Part model, mm, in its own coordinate system. Face numbers are marked on the shaded views. Round coordinates to 2 decimals unless told otherwise and drop trailing zeros. Write each loop counter-clockwise with the first axis right and the second up, starting at its lowest first coordinate (ties: lowest second). Pieces come first, ordered by that corner, then holes. Notation, with made-up numbers: M 67.5,-17 L 112.5,-17 A18 cw 112.5,-12 Z; hole C 25,2.5 d11. An arc over 180 degrees is marked long. Use a Markdown table: item, result. Add a question column.
1) Wall check: probe 1 along X at (y, z) = (0, 1.35); probe 2 along X at (y, z) = (-5.25, 0.75). Give the ranges that are in metal, low to high.
2) Two-plate mould, pull along Y, no slides. Class the marked faces 1, 2 and 3: released by +Y, released by -Y, zero draft, split by the parting line, or undercut.
3) Slice it at C-C on z = -1.05. Write the cut outline in (x, y), plus the area to 3 significant figures.
4) Drop flat-ended pins along their axis: P1, Ø7, axis at x = 0, y = 0, coming from the +Z side; P2, Ø2, axis at y = 4.5, z = 0, coming from the +X side; P3, Ø3, axis at x = -6, z = -2, coming from the -Y side. Give the stop position or say it passes through.
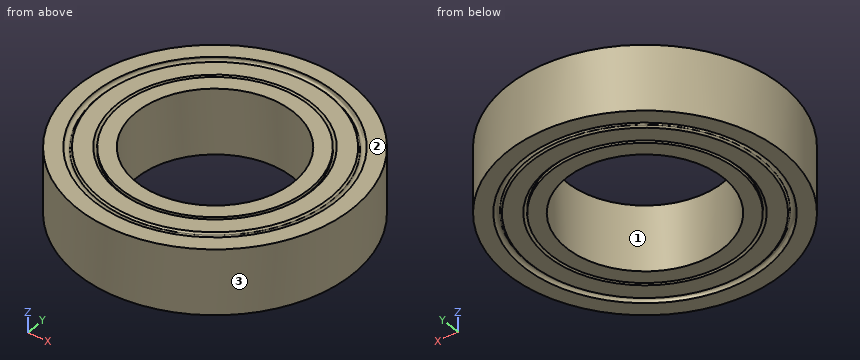
Autodesk Inventor part; units mm, degrees
ref_plane "YZ Plane" through (0, 0, 0) normal (1, 0, 0) x (0, 1, 0)
ref_plane "XZ Plane" through (0, 0, 0) normal (0, 1, 0) x (-1, 0, 0)
ref_plane "XY Plane" through (0, 0, 0) normal (0, 0, 1) x (1, 0, 0)
sketch "Эскиз1" plane through (0, 0, 0) normal (1, 0, 0) x (0, 1, 0)
  line L0 (6, -2.5) -> (6, 2.5)
  line L1 (10.5, 2.5) -> (10.5, -2.5)
  arc A0 (8.8667, 2.3707) -> (9.2616, 2.5) centre (9.0853, 2.3707) ccw
  line L2 (8.8667, 2.3707) -> (8.7374, 2.5)
  line L3 (8.8667, 2.3707) -> (9.0495, 2.3707) construction
  line L4 (7.4323, 2.5) -> (7.196, 2.2638)
  line L5 (7.4323, 2.5) -> (7.8016, 2.5) construction
  line L6 (9.2616, 2.5) -> (10.5, 2.5)
  line L7 (6, 2.5) -> (7.196, 2.5)
  line L8 (7.4323, 2.5) -> (8.7374, 2.5)
  line L9 (7.196, 2.5) -> (7.196, 2.2638)
  line L10 (9.696, 0) -> (8.6749, 0)
  arc A1 (9.2616, -2.5) -> (8.8667, -2.3707) centre (9.0853, -2.3707) ccw
  line L11 (8.8667, -2.3707) -> (8.7374, -2.5)
  line L12 (8.8667, -2.3707) -> (9.0495, -2.3707) construction
  line L13 (7.4323, -2.5) -> (7.196, -2.2638)
  line L14 (7.4323, -2.5) -> (7.8016, -2.5) construction
  line L15 (9.2616, -2.5) -> (10.5, -2.5)
  line L16 (6, -2.5) -> (7.196, -2.5)
  line L17 (7.4323, -2.5) -> (8.7374, -2.5)
  line L18 (7.196, -2.5) -> (7.196, -2.2638)
  line L19 (10.5, -2.5) -> (9.2616, -2.5)
  line L20 (8.7374, -2.5) -> (7.4323, -2.5)
  line L21 (7.196, -2.5) -> (6, -2.5)
  line L22 (0, -3.5047) -> (0, 3.5047)
  point P0 (0, 0)
  point P1 (9.304, 2.5)
  point P2 (9.304, -2.5)
  dimension "d0" = 5
  dimension "d1" = 4.5
  dimension "d2" = 6
  dimension "d5" = 135
  dimension "d6" = 135
revolve "Вращение1" add sketch "Эскиз1" angle 360 about axis through (0, 0, -10) along (0, 0, 1)
properties part number "wheel bearing"
Entries:
| question | item | result |
|---|---|---|
| 1 | probe 1 | x = -10.5 to -6, 6 to 10.5 |
| 1 | probe 2 | x = -9.09 to -2.9, 2.9 to 9.09 |
| 2 | face 1 | undercut |
| 2 | face 2 | zero draft |
| 2 | face 3 | split by the parting line |
| 3 | outline | C 0,0 d21; hole C 0,0 d12 |
| 3 | area | 233 mm^2 |
| 4 | P1 | passes through |
| 4 | P2 | stops at x = 9.9 |
| 4 | P3 | stops at y = -9.49 |
